Check sheet for the modelled part. Datum: model origin and axes. Units: mm. Face numbers are marked on the shaded views. A direction names the side the tool comes from. Round coordinates to 2 decimals unless told otherwise and drop trailing zeros. Order: outer loops, then holes, each group sorted by start corner. A loop starts at its lowest first (then second) coordinate and runs counter-clockwise, first axis right, second up.
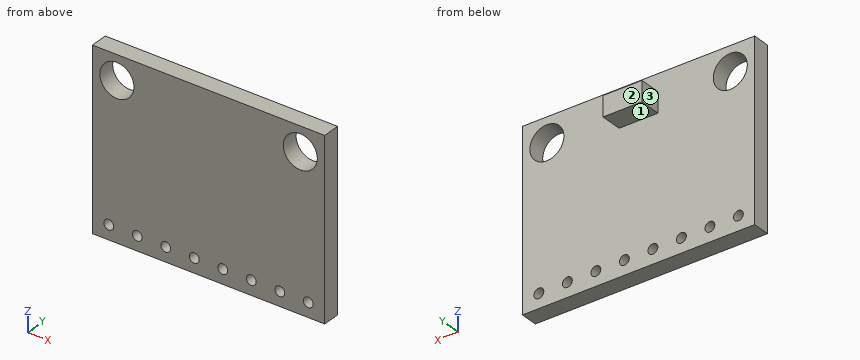
```python
from build123d import *

# Parameters (mm, degrees)
SKETCH1_W           = 20.45
SKETCH1_H           = 15.65
SKETCH1_R           = 1.5
SKETCH1_R_2         = 0.435
BOSS_EXTRUDE1_DEPTH = 1.524
SKETCH2_W           = 3.429
SKETCH2_H           = 1.778
BOSS_EXTRUDE2_DEPTH = 1.905


with BuildPart() as part:
    # Sketch1 → Boss-Extrude1 (new body)
    with BuildSketch(Plane(origin=(0, 0, 0), x_dir=(1, 0, 0), z_dir=(0, 1, 0))):
        with Locations((10.225, 7.825)):
            Rectangle(SKETCH1_W, SKETCH1_H)
        with Locations((2.15, 2.15)):
            Circle(SKETCH1_R, mode=Mode.SUBTRACT)
        with Locations((18.3, 2.15)):
            Circle(SKETCH1_R, mode=Mode.SUBTRACT)
        with Locations((1.435, 14.385)):
            Circle(SKETCH1_R_2, mode=Mode.SUBTRACT)
        with Locations((8.965, 14.385)):
            Circle(SKETCH1_R_2, mode=Mode.SUBTRACT)
        with Locations((6.455, 14.385)):
            Circle(SKETCH1_R_2, mode=Mode.SUBTRACT)
        with Locations((13.985, 14.385)):
            Circle(SKETCH1_R_2, mode=Mode.SUBTRACT)
        with Locations((11.475, 14.385)):
            Circle(SKETCH1_R_2, mode=Mode.SUBTRACT)
        with Locations((3.945, 14.385)):
            Circle(SKETCH1_R_2, mode=Mode.SUBTRACT)
        with Locations((16.495, 14.385)):
            Circle(SKETCH1_R_2, mode=Mode.SUBTRACT)
        with Locations((19.005, 14.385)):
            Circle(SKETCH1_R_2, mode=Mode.SUBTRACT)
    extrude(amount=BOSS_EXTRUDE1_DEPTH)

    # Sketch2 → Boss-Extrude2 (add)
    with BuildSketch(Plane(origin=(0, 1.524, 0), x_dir=(1, 0, 0), z_dir=(0, 1, 0))):
        with Locations((10.225, 2.391364263)):
            Rectangle(SKETCH2_W, SKETCH2_H)
    extrude(amount=BOSS_EXTRUDE2_DEPTH)


solid = part.part
```
Item 1: Sectioned sample at A-A (x = 18.3). Record the cut outline in (y, z).
Answer:
outline: (0, -15.65) - (1.52, -15.65) - (1.52, -3.65) - (0, -3.65) - close; (0, -0.65) - (1.52, -0.65) - (1.52, 0) - (0, 0) - close
Item 2: Sectioned sample at C-C (y = 0.9). State how many separate pieces and enclosed holes the cut face has, and give its area (3 significant figures).
Answer:
separate pieces: 1
enclosed holes: 10
area: 301 mm2
Item 3: Sectioned sample at D-D (x = 10.5). Record the cut outline in (y, z), and give its area (3 significant figures).
Answer:
outline: (0, -15.65) - (1.52, -15.65) - (1.52, -3.28) - (3.43, -3.28) - (3.43, -1.5) - (1.52, -1.5) - (1.52, 0) - (0, 0) - close
area: 27.2 mm2
Item 4: Scan lines: line 1 along X through (y, z) = (0.9, -2.15); line 2 along Z through (x, y) = (2.15, 0.6); line 3 along Z through (x, y) = (14, 1.1). Record each from-to range of solid material in increasing order.
Answer:
line 1: x = 0 to 0.65, 3.65 to 16.8, 19.8 to 20.45
line 2: z = -15.65 to -3.65, -0.65 to 0
line 3: z = -15.65 to -14.82, -13.95 to 0
Item 5: Access from +Z, -Z, +X, -X, +Y, -Y to the whole of each face (thin tool, end or side, straight path). Record for the marked faces 1, 2 and 3.
Answer:
face 1: -Z, +X, -X, +Y
face 2: +Z, -Z, +X, -X, +Y
face 3: +Z, -Z, -X, +Y
Item 6: Go/stop test with flat-tipped pins: P1, Ø1.5, axis at x = 9.5, y = 2.5, coming from the -Z side; P2, Ø0.5, axis at y = 2.5, z = -3, coming from the -X side. Record where each tip stops, or that it passes through.
Answer:
P1: stops at z = -3.28
P2: stops at x = 8.51
Item 7: Sectioned sample at B-B (z = -2.15). Record the cut outline in (x, y).
Answer:
outline: (0, 0) - (0.65, 0) - (0.65, 1.52) - (0, 1.52) - close; (3.65, 0) - (16.8, 0) - (16.8, 1.52) - (11.94, 1.52) - (11.94, 3.43) - (8.51, 3.43) - (8.51, 1.52) - (3.65, 1.52) - close; (19.8, 0) - (20.45, 0) - (20.45, 1.52) - (19.8, 1.52) - close
